Here's how the part is built. I have some questions about the finished solid (model axes, mm). A direction names the side the tool comes from. Coordinates: 2 decimals unless noted, no trailing zeros. Write each loop counter-clockwise with the first axis right and the second up, starting at its lowest first coordinate (ties: lowest second). Pieces come first, ordered by that corner, then holes. Notation, with made-up numbers: (31, 43.25) - (60, 43.25) arc R21 ccw to (60, 80.25) - close; hole circle Ø9 at (16.25, 39). An arc over 180 degrees is marked (long way). Answer in a Markdown table with one row per item. Add a question column.
Item 1: I'm going to push flat-ended pins straight in: pin 1 (3 mm diameter, centred on y = 79, z = 28, fed in from +X); pin 2 (12 mm diameter, centred on x = -40.5, y = 17.5, fed in from -Z); pin 3 (9 mm diameter, centred on x = -38.36, z = 47.49, fed in from +Y); pin 4 (18.5 mm diameter, centred on x = -12, z = 18.5, fed in from -Y). Where does each tip first touch, or does it pass through?
Item 2: If I drill on probe 1 along Y at (x, z) = (-11, 15); probe 2 along Y at (x, z) = (-15, 59); probe 3 along Z at (x, y) = (-16, 21), over which ranges is the centre line in solid material (lowest first)? Write a range as from..to.
Item 3: Which directions (+Z, -Z, +X, -X, +Y, -Y) give clear straight access to the entire face, cutting with the end or side of a thin tool? Please do faces 1 (the face through (-22, 50, 18)), 2 (the face through (-23.67, 6.141, 31.123)), 3 (the face through (-33, 5, 42)), 4 (the face through (-11.522, 6.972, 55.373)), 5 (the face through (-21, 2, 59)).
Item 4: Imagine slicing it at C-C (x = -33). Please give me the cut outline in (y, z).
Item 5: Imagine slicing it at D-D (z = 47.5). Please give me the cut outline in (x, y).
Item 6: We'd pull the mould along X, two halves only. Please class faces 6 (the face through (-38.242, 2.465, 44.743)), 7 (the face through (-18, 40, 29.921)), 8 (the face through (-2.071, 79, 28)): +X half, -X half, draft (parallel to the pull), parting line (faces both ways), or undercut.
Item 7: Imagine slicing it at B-B (y = 57.5). Please give me the cut outline in (x, z), plus the area to 3 significant figures.
Item 8: Imagine slicing it at A-A (z = 21.5). Please give me the cut outline in (x, y), plus the area to 3 significant figures.
from build123d import *

# Parameters (mm, degrees)
SKETCH1_R           = 2.75
BOSS_EXTRUDE1_DEPTH = 50
SKETCH2_R           = 2.2
BOSS_EXTRUDE2_DEPTH = 5
BOSS_EXTRUDE3_DEPTH = 32
SKETCH4_W           = 31.007197848
SKETCH4_H           = 89.787861365
CUT_EXTRUDE1_DEPTH  = 5
FILLET2_R           = 3
SKETCH6_W           = 76.819231413
SKETCH6_H           = 36.721827539
CUT_EXTRUDE2_DEPTH  = 45
FILLET3_R           = 4
SKETCH7_W           = 24
SKETCH7_H           = 3
BOSS_EXTRUDE4_DEPTH = 30
BOSS_EXTRUDE5_DEPTH = 4
SKETCH9_W           = 70
SKETCH9_H           = 5
CUT_EXTRUDE3_DEPTH  = 30
BOSS_EXTRUDE6_DEPTH = 36


with BuildPart() as part:
    # Sketch1 → Boss-Extrude1 (new body)
    with BuildSketch(Plane(origin=(0, 0, 0), x_dir=(1, 0, 0), z_dir=(0, 1, 0))):
        Polygon((-48.36251287, -26.4206039), (-13.721496719, -26.4206039), (12.928503281, -26.4206039), (12.928503281, -29.9206039), (-0.731115662, -29.9206039), (-48.36251287, -57.4206039), align=None)
        with Locations(Location((-21.908030198, -37.990095825, 0), (0, 0, 270))):
            Circle(SKETCH1_R, mode=Mode.SUBTRACT)
        with Locations(Location((-38.36251287, -47.490095825, 0), (0, 0, 270))):
            Circle(SKETCH1_R, mode=Mode.SUBTRACT)
    extrude(amount=BOSS_EXTRUDE1_DEPTH)

    # Sketch2 → Boss-Extrude2 (add)
    with BuildSketch(Plane(origin=(0, 50, 0), x_dir=(1, 0, 0), z_dir=(0, 1, 0))):
        Polygon((-48.36251287, -26.4206039), (12.928503281, -26.4206039), (12.928503281, -4.4206039), (1.63748713, -4.4206039), (1.63748713, -11.9206039), (-48.36251287, -11.9206039), align=None)
        with Locations(Location((-37.46251287, -15.6206039, 0), (0, 0, 270))):
            Circle(SKETCH2_R, mode=Mode.SUBTRACT)
    extrude(amount=-BOSS_EXTRUDE2_DEPTH)

    # Sketch3 → Boss-Extrude3 (add)
    with BuildSketch(Plane(origin=(0, 50, 0), x_dir=(1, 0, 0), z_dir=(0, 1, 0))):
        Polygon((12.928503281, -4.4206039), (9.028503281, -4.4206039), (9.028503281, -25.9206039), (-48.36251287, -25.9206039), (-48.36251287, -29.9206039), (6.778503281, -29.9206039), (12.928503281, -29.9206039), align=None)
    extrude(amount=BOSS_EXTRUDE3_DEPTH)

    # Sketch4 → Cut-Extrude1 (cut)
    with BuildSketch(Plane(origin=(0, 0, 4.4206039), x_dir=(-1, 0, 0), z_dir=(0, 0, -1))):
        with Locations((-11.123097368, 55.483744722)):
            Rectangle(SKETCH4_W, SKETCH4_H)
    extrude(amount=-CUT_EXTRUDE1_DEPTH, mode=Mode.SUBTRACT)

    # Fillet2
    fillet2_edges = [part.edges().sort_by_distance(p)[0] for p in [
        (-19.667004794, 50, 25.9206039),
        (9.028503281, 50, 17.6706039),
    ]]
    fillet(fillet2_edges, radius=FILLET2_R)

    # Sketch6 → Cut-Extrude2 (cut)
    with BuildSketch(Plane(origin=(0, 50, 0), x_dir=(1, 0, 0), z_dir=(0, 1, 0))):
        with Locations((-17.852673028, -48.28151767)):
            Rectangle(SKETCH6_W, SKETCH6_H)
    extrude(amount=-CUT_EXTRUDE2_DEPTH, mode=Mode.SUBTRACT)

    # Fillet3
    fillet3_edges = [part.edges().sort_by_distance(p)[0] for p in [
        (-0.731115662, 2.5, 29.9206039),
        (-48.36251287, 2.5, 57.4206039),
        (-24.546814266, 5, 29.9206039),
    ]]
    fillet(fillet3_edges, radius=FILLET3_R)

    # Sketch7 → Boss-Extrude4 (add)
    with BuildSketch(Plane(origin=(12.773222622, 0, 22.123870557), x_dir=(0.8660254037844415, 0, -0.49999999999999506), z_dir=(0.49999999999999506, 0, 0.8660254037844415))):
        with Locations((-47.665263456, 3.5)):
            Rectangle(SKETCH7_W, SKETCH7_H)
    extrude(amount=BOSS_EXTRUDE4_DEPTH)

    # Sketch8 → Boss-Extrude5 (add)
    with BuildSketch(Plane(origin=(0, 5, 0), x_dir=(1, 0, 0), z_dir=(0, 1, 0))):
        Polygon((-18.113801564, -39.956502285), (-38.898411255, -51.956502285), (-23.898411255, -77.937264399), (-3.113801564, -65.937264399), align=None)
        Polygon((-23.666360447, -74.339188187), (-6.345852372, -64.339188187), (-16.845852372, -46.152654708), (-34.166360447, -56.152654708), align=None, mode=Mode.SUBTRACT)
    extrude(amount=BOSS_EXTRUDE5_DEPTH)

    # Sketch9 → Cut-Extrude3 (cut)
    with BuildSketch(Plane.XY.offset(29.9206039)):
        with Locations((-13.36251287, 79.5)):
            Rectangle(SKETCH9_W, SKETCH9_H)
    extrude(amount=-CUT_EXTRUDE3_DEPTH, mode=Mode.SUBTRACT)

    # Sketch11 → Boss-Extrude6 (add)
    with BuildSketch(Plane(origin=(0, 45, 0), x_dir=(1, 0, 0), z_dir=(0, 1, 0))):
        Polygon((7.928503281, -29.9206039), (-2.071496719, -29.9206039), (-2.071496719, -27.9206039), (-2.071496719, -25.9206039), (7.928503281, -25.9206039), align=None)
    extrude(amount=BOSS_EXTRUDE6_DEPTH)


solid = part.part
Here are the results:
| question | item | result |
|---|---|---|
| 1 | pin 1 | stops at x = 7.93 |
| 1 | pin 2 | stops at z = 26.42 |
| 1 | pin 3 | stops at y = 9 |
| 1 | pin 4 | stops at y = 0 |
| 2 | probe 1 | y = 45..50 |
| 2 | probe 2 | y = 2..5 |
| 2 | probe 3 | z = 26.42..29.92 |
| 3 | face 1 | -Z, -X, +Y |
| 3 | face 2 | +X, -X, +Y |
| 3 | face 3 | -X, +Y |
| 3 | face 4 | +Y |
| 3 | face 5 | +Z, +X, -Y |
| 4 | outline | (0, 26.42) - (45, 26.42) - (45, 11.92) - (50, 11.92) - (50, 22.92) arc R3 cw to (53, 25.92) - (77, 25.92) - (77, 29.92) - (9, 29.92) arc R4 cw to (5, 33.92) - (5, 48.55) - (9, 48.55) - (9, 55.48) - (5, 55.48) - (5, 58.17) - (9, 58.17) - (9, 62.17) - (2, 62.17) - (2, 48.55) - (0, 48.55) - close |
| 5 | outline | (-48.36, 0) - (-41.11, 0) - (-41.11, 5) - (-48.36, 5) - close; (-35.61, 0) - (-31.18, 0) - (-31.18, 2) - (-13.76, 2) - (-13.76, 9) - (-16.07, 9) - (-16.07, 5) - (-19.18, 5) - (-19.18, 9) - (-31.18, 9) - (-31.18, 5) - (-35.61, 5) - close |
| 6 | face 6 | undercut |
| 6 | face 7 | draft |
| 6 | face 8 | -X half |
| 7 | outline | (-48.36, 25.92) - (9.03, 25.92) - (9.03, 9.42) - (12.93, 9.42) - (12.93, 29.92) - (-48.36, 29.92) - close |
| 7 | area | 310 mm2 |
| 8 | outline | (-48.36, 45) - (12.93, 45) - (12.93, 77) - (9.03, 77) - (9.03, 53) arc R3 cw to (6.03, 50) - (-48.36, 50) - close |
| 8 | area | 414 mm2 |
